Model file for the job. Use its own axes, mm. Face numbers are marked on the shaded views. A direction names the side the tool comes from. Round coordinates to 2 decimals unless told otherwise and drop trailing zeros. Loops run counter-clockwise (first coordinate to the right, second up) from the corner with the lowest first, then second, coordinate; pieces in that order, holes last. Notation, with made-up numbers: (-11, 22.25) - (28, 22.25) arc R19 cw to (28, 53.25) - close; hole circle Ø11 at (10, 5). An arc over 180 degrees is marked (long way). Answer as a JSON object with one key per item and string values.
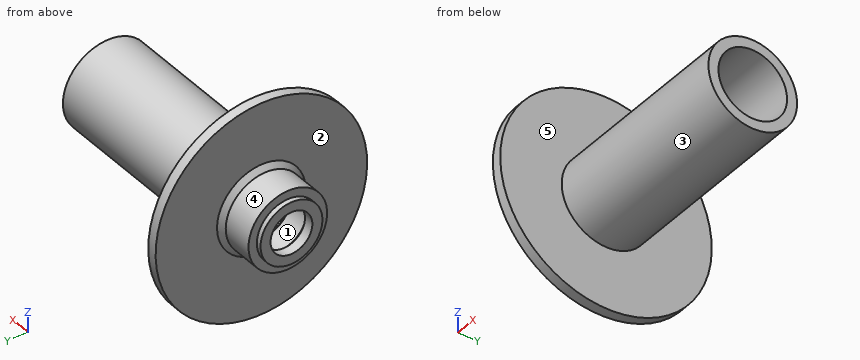
from build123d import *

# Parameters (mm, degrees)
SKETCH2_W = 1.2
SKETCH2_H = 7.341985405


# Read off the part's stored shape, not the designer's step: Revolve-Thin1
with BuildPart() as part:
    # Revolve-Thin1 outline → Revolve-Thin1 (revolve)
    with BuildSketch(Plane.YX):
        Polygon((4.1, 5.4), (3.5, 4.8), (3.5, 1.8), (3.1, 1.8), (2.5, 1.2), (2.5, 0), (3.7, 0), (3.7, 0.6), (4.7, 0.6), (4.7, 4.302943725), (5.3, 4.902943725), (5.3, 30), (4.1, 30), align=None)
    revolve(axis=Axis((0, 0, 0), (1, 0, 0)))

    # Sketch2 → Revolve-Thin2 (revolve)
    with BuildSketch(Plane.XY, mode=Mode.PRIVATE) as revolve_thin2_sk:
        with Locations((5.502943725, 8.970992703)):
            Rectangle(SKETCH2_W, SKETCH2_H)
    revolve(revolve_thin2_sk.sketch.rotate(Axis((0, 0, 0), (1, 0, 0)), 90), axis=Axis((0, 0, 0), (1, 0, 0)))


solid = part.part
1) Slice it at D-D on y = 11.25. List the corners of the cut face in (x, z), then the cut area to 3 significant figures.
Values follow:
{"outline": "(4.9, -5.77) - (6.1, -5.77) - (6.1, 5.77) - (4.9, 5.77) - close", "area": "13.8 mm²"}
2) Two-plate mould, pull along Z, no slides. Class the marked faces 1, 2 and 3: pulls with the +Z half, pulls with the -Z half, needs draft (parallel to the pull), parting line crosses it, or undercut.
Values follow:
{"face 1": "undercut", "face 2": "needs draft", "face 3": "parting line crosses it"}
3) Probe probe 1 along Z at (x, y) = (13, -0.25); probe 2 along Z at (x, y) = (0.45, 0); probe 3 along X at (y, z) = (0.75, -8.5). List the from-to ranges inside material, lowest first.
Values follow:
{"probe 1": "-5.29 to -4.09, 4.09 to 5.29", "probe 2": "-3.7 to -2.5, 2.5 to 3.7", "probe 3": "4.9 to 6.1"}
4) Drop flat-ended pins along their axis: P1, Ø4.5, axis at y = 0, z = 0, coming from the -X side; P2, Ø12, axis at x = 5, z = 6, coming from the +Y side; P3, Ø8, axis at x = 22.5, y = -3, coming from the -Z side; P4, Ø5, axis at x = 13, z = -1.5, coming from the -Y side. Give the stop position or say it passes through.
Values follow:
{"P1": "through", "P2": "y = 12.64", "P3": "z = -5.3", "P4": "y = -5.3"}
5) Tool access for the marked faces 4 and 5: list every direction of +Z, -Z, +X, -X, +Y, -Y with a clear straight run to the whole face (end or side of a thin tool).
Values follow:
{"face 4": "-X", "face 5": "+X"}
6) Slice it at C-C on x = 10.5. List the corners of the cut face in (y, z), then the cut area to 3 significant figures.
Values follow:
{"outline": "circle Ø10.6 at (0, 0); hole circle Ø8.2 at (0, 0)", "area": "35.4 mm²"}
